from build123d import *

# Parameters (mm, degrees)
BOSS_EXTRUDE1_DEPTH   = 152.4
SKETCH1_W             = 228.6
SKETCH1_H             = 6.35
BOSS_EXTRUDE1_2_DEPTH = 152.4
SKETCH3_W             = 647.7
SKETCH3_H             = 209.55
BOSS_EXTRUDE2_DEPTH   = 0.635


with BuildPart() as part:
    # Sketch1 → Boss-Extrude1 (new body)
    with BuildSketch(Plane.XY):
        Polygon((-94.045128316, 6.35), (566.354871684, 6.35), (566.354871684, -209.55), (560.004871684, -209.55), (560.004871684, 0), (-87.695128316, 0), (-87.695128316, -209.55), (-94.045128316, -209.55), align=None)
    extrude(amount=BOSS_EXTRUDE1_DEPTH)



with BuildPart() as body_2:
    # Sketch1 → Boss-Extrude1 2 (new body)
    with BuildSketch(Plane.XY):
        with Locations((242.504871684, -206.375)):
            Rectangle(SKETCH1_W, SKETCH1_H)
    extrude(amount=BOSS_EXTRUDE1_2_DEPTH)


with BuildPart() as part_1:
    add(part.part)

    add(body_2.part)  # Boss-Extrude2 merges body 2
    # Sketch3 → Boss-Extrude2 (add)
    with BuildSketch(Plane(origin=(0, 0, 0), x_dir=(-1, 0, 0), z_dir=(0, 0, -1))):
        with Locations((-236.154871684, -104.775)):
            Rectangle(SKETCH3_W, SKETCH3_H)
    extrude(amount=-BOSS_EXTRUDE2_DEPTH)


solid = part_1.part
Input: part model. Units: mm. Frame: model coordinates. A direction names the side the tool comes from. Coordinates: 2 decimals unless noted, no trailing zeros. Loops run counter-clockwise (first coordinate to the right, second up) from the corner with the lowest first, then second, coordinate; pieces in that order, holes last. Notation, with made-up numbers: (-20.5, 46) -> (-4.5, 46) arc R22 cw to (-4.5, 71) -> close; hole circle Ø3 at (30.25, 35.5). An arc over 180 degrees is marked (long way). Write item = value, one per line. Start each with the question number.
Item 1: Cut plane B-B, the plane x = 371. Return loops of the section in (y, z) (3 decimals), plus the area to 3 significant figures.
Item 2: Reachability of faces 5 (the face through (238, -209.55, 70)), 6 (the face through (-87.695, -103, 75)) from +Z, -Z, +X, -X, +Y, -Y: full face, straight path, thin tool, end or side. Return the list, or none.
Item 3: Cut plane C-C, the plane y = -147.5. Return loops of the section in (x, z) (3 decimals).
Item 4: Cut plane D-D, the plane x = 291. Return loops of the section in (y, z) (3 decimals), plus the area to 3 significant figures.
Item 5: First-contact query: P1, Ø8, axis at x = 120, z = 131, coming from the -Y side. Flat tip, straight axial feed; report the tip coordinate or a pass-through.
Item 6: Mould query, pull axis Y, two halves, no side actions, for faces 1 (the face through (241, -203.2, 75)), 2 (the face through (238, 3, 152.4)), 3 (the face through (232, 6.35, 75)), 4 (the face through (241, 0, 75)). Classes: pulls with the +Y half, pulls with the -Y half, needs draft (parallel to the pull), parting line crosses it, or undercut.
Item 7: Material intervals for line 1 (X direction, y = -107, z = 65); line 2 (Y direction, x = 160, z = 65); line 3 (Z direction, x = 32.5, y = -86) (3 decimals), sorted ascending.
Item 8: Cut plane A-A, the plane z = 82. Return loops of the section in (x, y).
Ans:
q1.outline = (-209.55, 0) -> (6.35, 0) -> (6.35, 152.4) -> (0, 152.4) -> (0, 0.635) -> (-209.55, 0.635) -> close
q1.area = 1,100 mm²
q2.face_5 = +Z, -Z, +X, -X, -Y
q2.face_6 = +Z, -Y
q3.outline = (-94.045, 0) -> (566.355, 0) -> (566.355, 152.4) -> (560.005, 152.4) -> (560.005, 0.635) -> (-87.695, 0.635) -> (-87.695, 152.4) -> (-94.045, 152.4) -> close
q4.outline = (-209.55, 0) -> (6.35, 0) -> (6.35, 152.4) -> (0, 152.4) -> (0, 0.635) -> (-203.2, 0.635) -> (-203.2, 152.4) -> (-209.55, 152.4) -> close
q4.area = 2,060 mm²
q5.P1 = 0
q6.face_1 = undercut
q6.face_2 = needs draft
q6.face_3 = pulls with the +Y half
q6.face_4 = undercut
q7.line_1 = -94.05 to -87.7, 560 to 566.35
q7.line_2 = -209.55 to -203.2, 0 to 6.35
q7.line_3 = 0 to 0.635
q8.outline = (-94.05, -209.55) -> (-87.7, -209.55) -> (-87.7, 0) -> (560, 0) -> (560, -209.55) -> (566.35, -209.55) -> (566.35, 6.35) -> (-94.05, 6.35) -> close; (128.2, -209.55) -> (356.8, -209.55) -> (356.8, -203.2) -> (128.2, -203.2) -> close
